For this review, use the dimensioned drawing (mm, ordinates from the lowest corner) and the shaded views. A direction names the side the tool comes from. Round coordinates to 2 decimals unless told otherwise and drop trailing zeros. Loops run counter-clockwise (first coordinate to the right, second up) from the corner with the lowest first, then second, coordinate; pieces in that order, holes last. Notation, with made-up numbers: M -31,75 L -14,75 A16 cw -14,97 Z; hole C 63,-30.5 d11. An arc over 180 degrees is marked long. Answer as a JSON object with one key per item and string values. Group by question number.
Item 1: The part is to be moulded in two halves that separate along Y. For the marked faces 1, 2, 3 and 4, say which applies: +Y half, -Y half, draft (parallel to the pull), parting line (faces both ways), or undercut.
Item 2: Consider section D-D (x = 92). Give the boundary of the cut face in (y, z).
Item 3: To check wall thickness, follow line 1 (Y direction, x = 60, z = 22.75); line 2 (Y direction, x = 18.5, z = 14.25); line 3 (Y direction, x = 70, z = 18.25). State the ranges of each line that lie inside material, in increasing order.
Item 4: Consider section A-A (x = 60). Give the boundary of the cut face in (y, z).
Item 5: Insertion check: P1, Ø12, axis at y = 25, z = 20.5, coming from the +X side; P2, Ø1.5, axis at y = 8.5, z = 4.5, coming from the -X side; P3, Ø4, axis at y = 49.5, z = 4.5, coming from the +X side; P4, Ø10, axis at y = 21.5, z = 10, coming from the -X side. Each pin has a flat end and moves straight along its axis. Give the tip position at first contact, or say it passes through.
Item 6: Consider section C-C (y = 42). Give the boundary of the cut face in (x, z).
Item 7: Tool access review of the marked faces 5, 6 and 7: name each direction out of +Z, -Z, +X, -X, +Y, -Y from which nothing blocks a thin tool from reaching the whole face with its end or side.
Item 8: Consider section B-B (z = 16.5). Give the boundary of the cut face in (x, y).
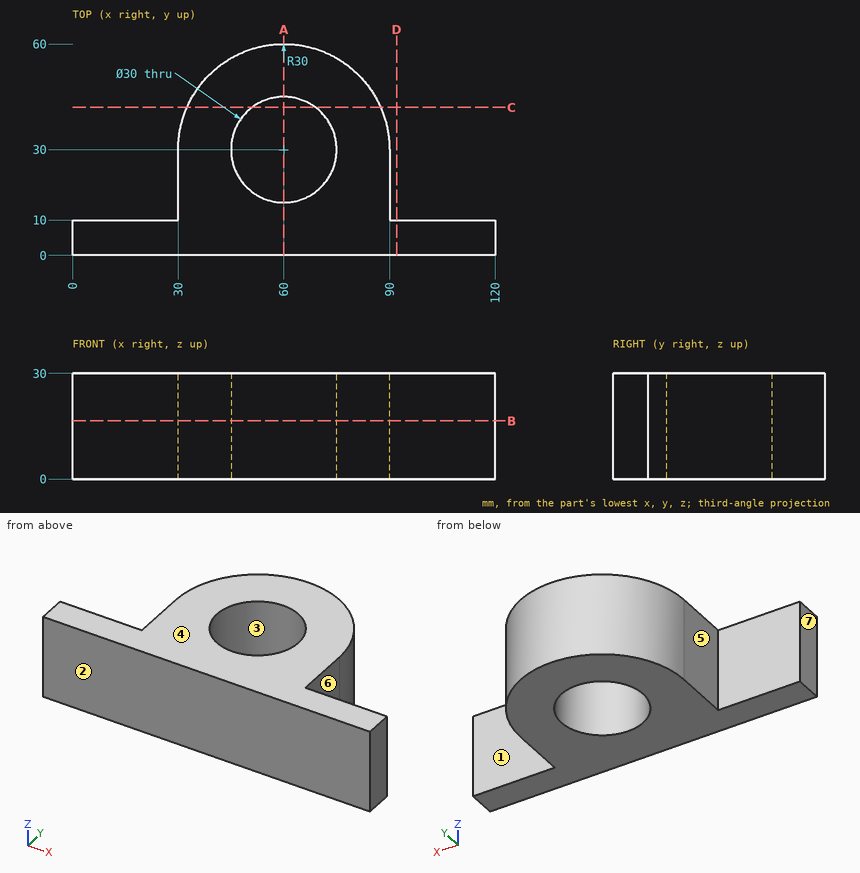
Geometry results:
{
 "1": {"face 1": "+Y half", "face 2": "-Y half", "face 3": "undercut", "face 4": "draft"},
 "2": {"outline": "M 0,0 L 10,0 L 10,30 L 0,30 Z"},
 "3": {"line 1": "y = 0 to 15, 45 to 60", "line 2": "y = 0 to 10", "line 3": "y = 0 to 18.82, 41.18 to 58.28"},
 "4": {"outline": "M 0,0 L 15,0 L 15,30 L 0,30 Z; M 45,0 L 60,0 L 60,30 L 45,30 Z"},
 "5": {"P1": "stops at x = 90", "P2": "stops at x = 0", "P3": "stops at x = 84.37", "P4": "stops at x = 30"},
 "6": {"outline": "M 32.5,0 L 51,0 L 51,30 L 32.5,30 Z; M 69,0 L 87.5,0 L 87.5,30 L 69,30 Z"},
 "7": {"face 5": "+Z, -Z, -X, +Y", "face 6": "+Z, -Z, +X, +Y", "face 7": "+Z, -Z, -X, +Y, -Y"},
 "8": {"outline": "M 0,0 L 120,0 L 120,10 L 90,10 L 90,30 A30 ccw 30,30 L 30,10 L 0,10 Z; hole C 60,30 d30"}
}
